Read the model definition and answer for the solid it produces. Units are mm, in the model's axes. Give positions to 0.01 mm unless a question says otherwise; leave off trailing zeros. Order: outer loops, then holes, each group sorted by start corner. A loop starts at its lowest first (then second) coordinate and runs counter-clockwise, first axis right, second up. Notation, with made-up numbers: (-32, 24) - (1, 24) arc R20 ccw to (1, 61) - close; hole circle Ø2 at (58.25, 48.25). An arc over 180 degrees is marked (long way). Answer as CSV lines item,"result". Start each with the question number.
from build123d import *

# Parameters (mm, degrees)
SKETCH086_W     = 445
SKETCH086_H     = 232
PAD026_DEPTH    = 3
SKETCH087_R     = 9.5
POCKET057_DEPTH = 5
FILLET011_R     = 2
POCKET058_DEPTH = 10.001
SKETCH089_R     = 6
SKETCH089_R_2   = 5
POCKET059_DEPTH = 5
POCKET064_DEPTH = 5


with BuildPart() as part:
    # Sketch086 → Pad026 (new body)
    with BuildSketch(Plane.XY):
        Rectangle(SKETCH086_W, SKETCH086_H)
    extrude(amount=PAD026_DEPTH)

    # Sketch087 (on Face6 of Pad026) → Pocket057 (cut)
    with BuildSketch(Plane.XY.offset(3)):
        with Locations((-183, 55)):
            Circle(SKETCH087_R)
        with Locations((-183, 33)):
            Circle(SKETCH087_R)
        with Locations((-183, 11)):
            Circle(SKETCH087_R)
        with Locations((-183, -11)):
            Circle(SKETCH087_R)
        with Locations((-183, -33)):
            Circle(SKETCH087_R)
        with Locations((-183, -55)):
            Circle(SKETCH087_R)
        with Locations((-164, 44)):
            Circle(SKETCH087_R)
        with Locations((-164, 22)):
            Circle(SKETCH087_R)
        with Locations((-164, 0)):
            Circle(SKETCH087_R)
        with Locations((-164, -22)):
            Circle(SKETCH087_R)
        with Locations((-164, -44)):
            Circle(SKETCH087_R)
        with Locations((-145, 55)):
            Circle(SKETCH087_R)
        with Locations((-145, 33)):
            Circle(SKETCH087_R)
        with Locations((-145, 11)):
            Circle(SKETCH087_R)
        with Locations((-145, -11)):
            Circle(SKETCH087_R)
        with Locations((-145, -33)):
            Circle(SKETCH087_R)
        with Locations((-145, -55)):
            Circle(SKETCH087_R)
        with Locations((-126, 44)):
            Circle(SKETCH087_R)
        with Locations((-126, 22)):
            Circle(SKETCH087_R)
        with Locations((-126, 0)):
            Circle(SKETCH087_R)
        with Locations((-126, -22)):
            Circle(SKETCH087_R)
        with Locations((-126, -44)):
            Circle(SKETCH087_R)
        with Locations((-107, 55)):
            Circle(SKETCH087_R)
        with Locations((-107, 33)):
            Circle(SKETCH087_R)
        with Locations((-107, 11)):
            Circle(SKETCH087_R)
        with Locations((-107, -11)):
            Circle(SKETCH087_R)
        with Locations((-107, -33)):
            Circle(SKETCH087_R)
        with Locations((-107, -55)):
            Circle(SKETCH087_R)
        with Locations((-88, -44)):
            Circle(SKETCH087_R)
        with Locations((-88, -22)):
            Circle(SKETCH087_R)
        with Locations((-88, 0)):
            Circle(SKETCH087_R)
        with Locations((-88, 22)):
            Circle(SKETCH087_R)
        with Locations((-88, 44)):
            Circle(SKETCH087_R)
        with Locations((-69, 55)):
            Circle(SKETCH087_R)
        with Locations((-69, 33)):
            Circle(SKETCH087_R)
        with Locations((-69, 11)):
            Circle(SKETCH087_R)
        with Locations((-69, -11)):
            Circle(SKETCH087_R)
        with Locations((-69, -33)):
            Circle(SKETCH087_R)
        with Locations((-50, 44)):
            Circle(SKETCH087_R)
        with Locations((-50, 22)):
            Circle(SKETCH087_R)
        with Locations((-50, 0)):
            Circle(SKETCH087_R)
        with Locations((-50, -22)):
            Circle(SKETCH087_R)
        with Locations((-50, -44)):
            Circle(SKETCH087_R)
        with Locations((-69, -55)):
            Circle(SKETCH087_R)
        with Locations((-31, 55)):
            Circle(SKETCH087_R)
        with Locations((-31, 33)):
            Circle(SKETCH087_R)
        with Locations((-31, 11)):
            Circle(SKETCH087_R)
        with Locations((-31, -11)):
            Circle(SKETCH087_R)
        with Locations((-31, -33)):
            Circle(SKETCH087_R)
        with Locations((-31, -55)):
            Circle(SKETCH087_R)
        with Locations((-12, -44)):
            Circle(SKETCH087_R)
        with Locations((-12, -22)):
            Circle(SKETCH087_R)
        with Locations((-12, 0)):
            Circle(SKETCH087_R)
        with Locations((-12, 22)):
            Circle(SKETCH087_R)
        with Locations((-12, 44)):
            Circle(SKETCH087_R)
        with Locations((7, 55)):
            Circle(SKETCH087_R)
        with Locations((7, 33)):
            Circle(SKETCH087_R)
        with Locations((7, 11)):
            Circle(SKETCH087_R)
        with Locations((7, -11)):
            Circle(SKETCH087_R)
        with Locations((7, -33)):
            Circle(SKETCH087_R)
        with Locations((7, -55)):
            Circle(SKETCH087_R)
        with Locations((26, -44)):
            Circle(SKETCH087_R)
        with Locations((26, -22)):
            Circle(SKETCH087_R)
        with Locations((26, 0)):
            Circle(SKETCH087_R)
        with Locations((26, 22)):
            Circle(SKETCH087_R)
        with Locations((26, 44)):
            Circle(SKETCH087_R)
        with Locations((45, 55)):
            Circle(SKETCH087_R)
        with Locations((45, 33)):
            Circle(SKETCH087_R)
        with Locations((45, 11)):
            Circle(SKETCH087_R)
        with Locations((45, -11)):
            Circle(SKETCH087_R)
        with Locations((64, 0)):
            Circle(SKETCH087_R)
        with Locations((64, 22)):
            Circle(SKETCH087_R)
        with Locations((64, 44)):
            Circle(SKETCH087_R)
        with Locations((45, -33)):
            Circle(SKETCH087_R)
        with Locations((45, -55)):
            Circle(SKETCH087_R)
        with Locations((64, -44)):
            Circle(SKETCH087_R)
        with Locations((64, -22)):
            Circle(SKETCH087_R)
        with Locations((83, 55)):
            Circle(SKETCH087_R)
        with Locations((83, 33)):
            Circle(SKETCH087_R)
        with Locations((83, 11)):
            Circle(SKETCH087_R)
        with Locations((83, -11)):
            Circle(SKETCH087_R)
        with Locations((83, -33)):
            Circle(SKETCH087_R)
        with Locations((83, -55)):
            Circle(SKETCH087_R)
        with Locations((102, 44)):
            Circle(SKETCH087_R)
        with Locations((102, 22)):
            Circle(SKETCH087_R)
        with Locations((102, 0)):
            Circle(SKETCH087_R)
        with Locations((102, -22)):
            Circle(SKETCH087_R)
        with Locations((102, -44)):
            Circle(SKETCH087_R)
        with Locations((121, 55)):
            Circle(SKETCH087_R)
        with Locations((121, 33)):
            Circle(SKETCH087_R)
        with Locations((121, 11)):
            Circle(SKETCH087_R)
        with Locations((121, -11)):
            Circle(SKETCH087_R)
        with Locations((121, -33)):
            Circle(SKETCH087_R)
        with Locations((121, -55)):
            Circle(SKETCH087_R)
        with Locations((140, 44)):
            Circle(SKETCH087_R)
        with Locations((140, 22)):
            Circle(SKETCH087_R)
        with Locations((140, 0)):
            Circle(SKETCH087_R)
        with Locations((140, -22)):
            Circle(SKETCH087_R)
        with Locations((140, -44)):
            Circle(SKETCH087_R)
        with Locations((159, 55)):
            Circle(SKETCH087_R)
        with Locations((159, 33)):
            Circle(SKETCH087_R)
        with Locations((159, 11)):
            Circle(SKETCH087_R)
        with Locations((159, -11)):
            Circle(SKETCH087_R)
        with Locations((159, -33)):
            Circle(SKETCH087_R)
        with Locations((159, -55)):
            Circle(SKETCH087_R)
        with Locations((-164, 66)):
            Circle(SKETCH087_R)
        with Locations((-126, 66)):
            Circle(SKETCH087_R)
        with Locations((-88, 66)):
            Circle(SKETCH087_R)
        with Locations((-50, 66)):
            Circle(SKETCH087_R)
        with Locations((-12, 66)):
            Circle(SKETCH087_R)
        with Locations((26, 66)):
            Circle(SKETCH087_R)
        with Locations((64, 66)):
            Circle(SKETCH087_R)
        with Locations((102, 66)):
            Circle(SKETCH087_R)
        with Locations((140, 66)):
            Circle(SKETCH087_R)
        with Locations((-164, -66)):
            Circle(SKETCH087_R)
        with Locations((-126, -66)):
            Circle(SKETCH087_R)
        with Locations((-88, -66)):
            Circle(SKETCH087_R)
        with Locations((-50, -66)):
            Circle(SKETCH087_R)
        with Locations((-12, -66)):
            Circle(SKETCH087_R)
        with Locations((26, -66)):
            Circle(SKETCH087_R)
        with Locations((64, -66)):
            Circle(SKETCH087_R)
        with Locations((102, -66)):
            Circle(SKETCH087_R)
        with Locations((140, -66)):
            Circle(SKETCH087_R)
        with Locations((178, 66)):
            Circle(SKETCH087_R)
        with Locations((178, 44)):
            Circle(SKETCH087_R)
        with Locations((178, 22)):
            Circle(SKETCH087_R)
        with Locations((178, 0)):
            Circle(SKETCH087_R)
        with Locations((178, -22)):
            Circle(SKETCH087_R)
        with Locations((178, -44)):
            Circle(SKETCH087_R)
        with Locations((178, -66)):
            Circle(SKETCH087_R)
    extrude(amount=-POCKET057_DEPTH, mode=Mode.SUBTRACT)

    # Fillet011
    fillet011_edges = [part.edges().sort_by_distance(p)[0] for p in [
        (-222.5, -116, 1.5),
        (222.5, -116, 1.5),
        (222.5, 116, 1.5),
        (-222.5, 116, 1.5),
    ]]
    fillet(fillet011_edges, radius=FILLET011_R)

    # Sketch088 → Pocket058 (cut, through all)
    with BuildSketch(Plane.XY.offset(10)):
        Polygon((188.873749, -62), (214.664444, -62), (214.664444, 62), (188.873749, 62), (188.873749, 11.724954), (183.462372, 4.250606), (183.462372, -4.752587), (188.873749, -11.972128), align=None)
    extrude(amount=-POCKET058_DEPTH, mode=Mode.SUBTRACT)

    # Sketch089 (on Face2 of Pocket058) → Pocket059 (cut)
    with BuildSketch(Plane(origin=(0, 0, 0), x_dir=(1, 0, 0), z_dir=(0, 0, -1))):
        with Locations((213.5, 50)):
            Circle(SKETCH089_R)
        with Locations((213.5, -50)):
            Circle(SKETCH089_R)
        with Locations((-213.5, 50)):
            Circle(SKETCH089_R)
        with Locations((-213.5, -50)):
            Circle(SKETCH089_R)
        with Locations((-163.5, 90)):
            Circle(SKETCH089_R_2)
        with Locations((-25.5, 90)):
            Circle(SKETCH089_R_2)
        with Locations((163.5, 90)):
            Circle(SKETCH089_R_2)
        with Locations((163.5, -90)):
            Circle(SKETCH089_R_2)
        with Locations((-25.5, -90)):
            Circle(SKETCH089_R_2)
        with Locations((-163.5, -90)):
            Circle(SKETCH089_R_2)
    extrude(amount=-POCKET059_DEPTH, mode=Mode.SUBTRACT)

    # Sketch095 (on Face5 of Pocket059) → Pocket064 (cut)
    with BuildSketch(Plane.XY.offset(3)):
        Polygon((-317.002441, 177.552841), (-30, 177.552841), (-30, -258.20929), (140, -258.20929), (140, 194.405518), (369.744232, 194.405518), (393.819366, -352.102783), (-350.707825, -320.203064), align=None)
    extrude(amount=-POCKET064_DEPTH, mode=Mode.SUBTRACT)


with BuildPart() as part_1:
    # Body022 placement: moved
    add(part.part.moved(Location((0, 0, -3))))


solid = part_1.part
(1) Flat-ended cylindrical pins translate along their axes: pin 1 Ø5 at (x, y) = (105.5, 4) entering from +Z; pin 2 Ø24.5 at (x, y) = (102, -44) entering from +Z. Find the tip coordinate at first contact, or state that the pin passes through.
(2) Section C-C, the plane y = 70 is taken. Write down the section's boundary in (x, z), and give its area (3 significant figures).
(3) Section B-B, the plane x = 102 is taken. State how many separate pieces and enclosed holes the cut face has, and give its area (3 significant figures).
(4) Determine the mould class of faces 1 (the cylindrical face through (130.502, -65.791, -1.479)), 2 (the cylindrical face through (-21.5, -11.19, -1.48)), 3 (the cylindrical face through (73.061, 46.854, -1.479)) for opening direction X: released by +X, released by -X, zero draft, split by the parting line, or undercut.
(5) Section A-A, the plane x = 45 is taken. Write down the section's boundary in (y, z).
(6) Straight lines are drawn through the part: line 1 (X direction, y = -68.5, z = -1.1); line 2 (X direction, y = 72, z = -2.25). For each, find the intervals that lie inside material, in ascending order. Write a range as [from, to].
Checks:
1,pin 1,"passes through"
1,pin 2,"stops at z = 0"
2,outline,"(-30, -3) - (-20.62, -3) - (-20.62, 0) - (-30, 0) - close; (-3.38, -3) - (17.38, -3) - (17.38, 0) - (-3.38, 0) - close; (34.62, -3) - (55.38, -3) - (55.38, 0) - (34.62, 0) - close; (72.62, -3) - (93.38, -3) - (93.38, 0) - (72.62, 0) - close; (110.62, -3) - (131.38, -3) - (131.38, 0) - (110.62, 0) - close"
2,area,"277 mm²"
3,separate pieces,"8"
3,enclosed holes,"0"
3,area,"297 mm²"
4,face 1,"released by +X"
4,face 2,"released by -X"
4,face 3,"undercut"
5,outline,"(-116, -3) - (-64.5, -3) - (-64.5, 0) - (-116, 0) - close; (-45.5, -3) - (-42.5, -3) - (-42.5, 0) - (-45.5, 0) - close; (-23.5, -3) - (-20.5, -3) - (-20.5, 0) - (-23.5, 0) - close; (-1.5, -3) - (1.5, -3) - (1.5, 0) - (-1.5, 0) - close; (20.5, -3) - (23.5, -3) - (23.5, 0) - (20.5, 0) - close; (42.5, -3) - (45.5, -3) - (45.5, 0) - (42.5, 0) - close; (64.5, -3) - (116, -3) - (116, 0) - (64.5, 0) - close"
6,line 1,"x = [-30, -21.17], [-2.83, 16.83], [35.17, 54.83], [73.17, 92.83], [111.17, 130.83]"
6,line 2,"x = [-30, -19.37], [-4.63, 18.63], [33.37, 56.63], [71.37, 94.63], [109.37, 132.63]"
